from build123d import *

# Parameters (mm, degrees)
F1_W     = 73
F1_H     = 73
F2_DEPTH = 16
F3_DEPTH = 2
F4_W     = 2
F4_H     = 73
F5_DEPTH = 14
F0_W     = 35.5
F0_H     = 23.5
F6_DEPTH = 2
F7_DEPTH = 2
F8_DEPTH = 16


with BuildPart() as f2:
    # F1 (on face) → F2 (new body)
    with BuildSketch(Plane.XY):
        Polygon((-38, 38), (-38, -38), (38, -38), (38, 38), (36.5, 38), (1, 38), (-1, 38), (-36.5, 38), align=None)
        Rectangle(F1_W, F1_H, mode=Mode.SUBTRACT)
    extrude(amount=F2_DEPTH)

    # F0 (on Top) → F3 (join)
    with BuildSketch(Plane.XY):
        Polygon((-38, -38), (38, -38), (38, 38), (36.5, 38), (1, 38), (-1, 38), (-36.5, 38), (-38, 38), align=None)
    extrude(amount=F3_DEPTH)

    # F4 (on face) → F5 (join)
    with BuildSketch(Plane.XY.offset(2)):
        Rectangle(F4_W, F4_H)
    extrude(amount=F5_DEPTH)

    # F0 (on Top) → F6 (join)
    with BuildSketch(Plane.XY):
        with Locations((-18.75, 49.75)):
            Rectangle(F0_W, F0_H)
    extrude(amount=F6_DEPTH)

    # F0 (on Top) → F7 (join)
    with BuildSketch(Plane.XY):
        with Locations((18.75, 49.75)):
            Rectangle(F0_W, F0_H)
    extrude(amount=F7_DEPTH)

    # F0 (on Top) → F8 (join)
    with BuildSketch(Plane.XY):
        Polygon((36.5, 38), (38, 38), (38, 63), (-38, 63), (-38, 38), (-36.5, 38), (-36.5, 61.5), (-1, 61.5), (-1, 38), (1, 38), (1, 61.5), (36.5, 61.5), align=None)
    extrude(amount=F8_DEPTH)


solid = f2.part
Model file for the job. Use its own axes, mm. A direction names the side the tool comes from. Give positions to 0.01 mm unless a question says otherwise; leave off trailing zeros. Loops run counter-clockwise (first coordinate to the right, second up) from the corner with the lowest first, then second, coordinate; pieces in that order, holes last. Notation, with made-up numbers: (20, -34.75) -> (67, -34.75) arc R18 cw to (67, -8.75) -> close; hole circle Ø7 at (-38, -36). An arc over 180 degrees is marked (long way). Use a Markdown table: item, result. Add a question column.
(1) Tool access for faces 1 (the flat face through (19, 38, 9)), 2 (the flat face through (-1, 13, 0)): list every direction of +Z, -Z, +X, -X, +Y, -Y with a clear straight run to the whole face (end or side of a thin tool).
(2) Drop flat-ended pins along their axis: pin 1 Ø1.5 at (x, y) = (-25, -8.5) entering from -Z; pin 2 Ø10.5 at (x, y) = (16, -11) entering from +Z. Give the stop position or say it passes through.
(3) Slice it at B-B on y = 51.5. List the corners of the cut face in (x, z), and give its area (3 significant figures).
(4) Slice it at A-A on x = 33.5. List the corners of the cut face in (y, z).
(5) Slice it at C-C on z = 11.5. List the corners of the cut face in (x, y), and give its area (4 significant figures).
(6) Wall check: line 1 along Y through (x, z) = (-13, 13.75); line 2 along X through (y, z) = (-33.5, 14.5); line 3 along Z through (x, y) = (-11, -28). Give the ranges that are in metal, low to high.
(7) Mould opens along Y. For faces 3 (the flat face through (19, -36.5, 9)), 4 (the flat face through (38, 12, 8)) say: +Y half, -Y half, draft (parallel to the pull), parting line (faces both ways), or undercut.
Filled sheet:
| question | item | result |
|---|---|---|
| 1 | face 1 | +Z |
| 1 | face 2 | -Z, +X, -X, +Y, -Y |
| 2 | pin 1 | z = 0 |
| 2 | pin 2 | z = 2 |
| 3 | outline | (-38, 0) -> (38, 0) -> (38, 16) -> (36.5, 16) -> (36.5, 2) -> (1, 2) -> (1, 16) -> (-1, 16) -> (-1, 2) -> (-36.5, 2) -> (-36.5, 16) -> (-38, 16) -> close |
| 3 | area | 222 mm2 |
| 4 | outline | (-38, 0) -> (63, 0) -> (63, 16) -> (61.5, 16) -> (61.5, 2) -> (38, 2) -> (38, 16) -> (36.5, 16) -> (36.5, 2) -> (-36.5, 2) -> (-36.5, 16) -> (-38, 16) -> close |
| 5 | outline | (-38, -38) -> (38, -38) -> (38, 63) -> (-38, 63) -> close; hole (-36.5, -36.5) -> (-1, -36.5) -> (-1, 36.5) -> (-36.5, 36.5) -> close; hole (-36.5, 38) -> (-1, 38) -> (-1, 61.5) -> (-36.5, 61.5) -> close; hole (1, -36.5) -> (36.5, -36.5) -> (36.5, 36.5) -> (1, 36.5) -> close; hole (1, 38) -> (36.5, 38) -> (36.5, 61.5) -> (1, 61.5) -> close |
| 5 | area | 824.5 mm2 |
| 6 | line 1 | -38 to -36.5, 36.5 to 38, 61.5 to 63 |
| 6 | line 2 | -38 to -36.5, -1 to 1, 36.5 to 38 |
| 6 | line 3 | 0 to 2 |
| 7 | face 3 | undercut |
| 7 | face 4 | draft |
